Geometry: final body of the model. Coordinates: model frame, mm. Face numbers are marked on the shaded views. A direction names the side the tool comes from. Round coordinates to 2 decimals unless told otherwise and drop trailing zeros. Loops run counter-clockwise (first coordinate to the right, second up) from the corner with the lowest first, then second, coordinate; pieces in that order, holes last. Notation, with made-up numbers: (20, 1) - (39, 1) arc R26 cw to (39, 31) - close; hole circle Ø6 at (-12, -28). An arc over 180 degrees is marked (long way). Use CSV: the item, a comma, the result in double quotes.
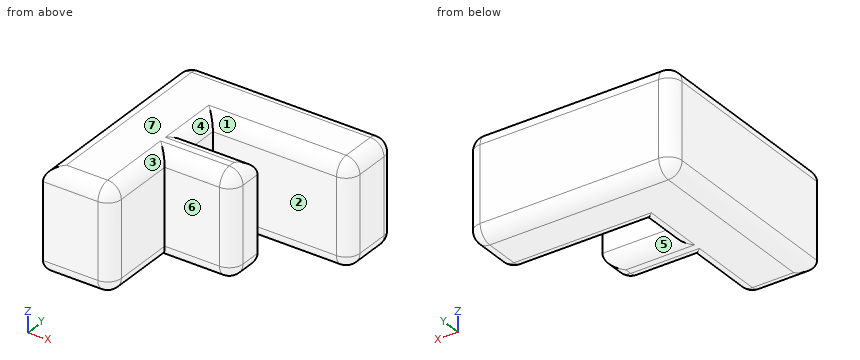
from build123d import *

# Parameters (mm, degrees)
F1_DEPTH = 15
F2_R     = 2


with BuildPart() as f1:
    # F0 (on Top) → F1 (new body)
    with BuildSketch(Plane.XY):
        Polygon((0, 30), (0, 0), (10, 0), (10, 11), (20, 11), (20, 16), (10, 16), (10, 21), (30, 21), (30, 30), align=None)
    extrude(amount=F1_DEPTH)

    # F2
    f2_edges = [f1.edges().sort_by_distance(p)[0] for p in [
        (30, 21, 7.5),
        (30, 30, 7.5),
        (30, 25.5, 0),
        (30, 25.5, 15),
        (20, 11, 7.5),
        (10, 0, 7.5),
        (20, 21, 0),
        (15, 30, 15),
        (0, 15, 0),
        (5, 0, 0),
        (10, 5.5, 0),
        (15, 11, 0),
        (20, 13.5, 0),
        (15, 16, 0),
        (10, 18.5, 0),
        (15, 30, 0),
        (0, 30, 7.5),
        (0, 15, 15),
        (5, 0, 15),
        (10, 5.5, 15),
        (15, 11, 15),
        (20, 13.5, 15),
        (15, 16, 15),
        (10, 18.5, 15),
        (20, 21, 15),
    ]]
    fillet(f2_edges, radius=F2_R)


solid = f1.part
Item 1: Section B-B on x = 21.25. Return the cut outline in (y, z).
Final values:
outline,"(21, 2) arc R2 ccw to (23, 0) - (28, 0) arc R2 ccw to (30, 2) - (30, 13) arc R2 ccw to (28, 15) - (23, 15) arc R2 ccw to (21, 13) - close"
Item 2: Section C-C on y = 18.75. Return the cut outline in (x, z), plus the area to 3 significant figures.
Final values:
outline,"(0, 2) arc R2 ccw to (2, 0) - (8, 0) arc R2 ccw to (10, 2) - (10, 13) arc R2 ccw to (8, 15) - (2, 15) arc R2 ccw to (0, 13) - close"
area,"147 mm²"
Item 3: Pin query (flat end, axial travel): P1, Ø2.5, axis at y = 18.5, z = 9, coming from the +X side; P2, Ø1.5, axis at x = 12, y = 4.5, coming from the +Z side; P3, Ø2, axis at y = 13, z = 13, coming from the +X side; P4, Ø9, axis at x = 15.5, z = 5.5, coming from the -Y side. Return the tip coordinate at first contact, or that it passes through.
Final values:
P1,"stops at x = 10"
P2,"passes through"
P3,"stops at x = 20"
P4,"stops at y = 11"
Item 4: Section A-A on z = 8.25. Return the cut outline in (x, y).
Final values:
outline,"(0, 0) - (8, 0) arc R2 ccw to (10, 2) - (10, 11) - (18, 11) arc R2 ccw to (20, 13) - (20, 16) - (10, 16) - (10, 21) - (28, 21) arc R2 ccw to (30, 23) - (30, 28) arc R2 ccw to (28, 30) - (2, 30) arc R2 ccw to (0, 28) - close"
Item 5: Material intervals for line 1 (Y direction, x = 12.75, z = 10.25); line 2 (X direction, y = 7, z = 9.25); line 3 (X direction, y = 13.5, z = 11.75), sorted ascending.
Final values:
line 1,"y = 11 to 16, 21 to 30"
line 2,"x = 0 to 10"
line 3,"x = 0 to 20"
Item 6: Mould query, pull axis Y, two halves, no side actions, for the marked faces 4, 5, 6 and 7. Classes: released by +Y, released by -Y, zero draft, split by the parting line, or undercut.
Final values:
face 4,"undercut"
face 5,"undercut"
face 6,"released by -Y"
face 7,"zero draft"
Item 7: Reachability of the marked faces 1, 2 and 3 from +Z, -Z, +X, -X, +Y, -Y: full face, straight path, thin tool, end or side. Return the list, or none.
Final values:
face 1,"+Z, +X"
face 2,"+Z, -Z, +X"
face 3,"+Z, +X, -Y"
Item 8: Section D-D on z = 1. Return the cut outline in (x, y), plus the area to 3 significant figures.
Final values:
outline,"(0.27, 0.27) - (8, 0.27) arc R1.73 ccw to (9.73, 2) - (9.73, 11.27) - (18, 11.27) arc R1.73 ccw to (19.73, 13) - (19.73, 15.73) - (9.73, 15.73) - (9.73, 21.27) - (28, 21.27) arc R1.73 ccw to (29.73, 23) - (29.73, 28) arc R1.73 ccw to (28, 29.73) - (2, 29.73) arc R1.73 ccw to (0.27, 28) - close"
area,"490 mm²"
